Check sheet for the modelled part. Datum: model origin and axes. Units: mm. Round coordinates to 2 decimals unless told otherwise and drop trailing zeros. Order: outer loops, then holes, each group sorted by start corner. A loop starts at its lowest first (then second) coordinate and runs counter-clockwise, first axis right, second up.
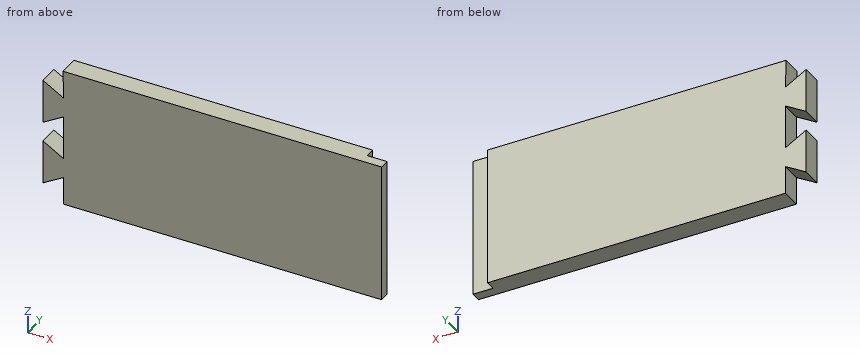
```python
from build123d import *

# Parameters (mm, degrees)
F0_W     = 340
F0_H     = 140
F1_DEPTH = 20
F4_DEPTH = 20
F2_W     = 10
F2_H     = 140
F5_DEPTH = 20


with BuildPart() as f1:
    # F0 (on Front) → F1 (new body)
    with BuildSketch(Plane.XZ):
        Rectangle(F0_W, F0_H)
    extrude(amount=F1_DEPTH)

    # F3 (on face) → F4 (cut)
    with BuildSketch(Plane(origin=(0, 0, 0), x_dir=(-1, 0, 0), z_dir=(0, 1, 0))):
        Polygon((149.1751, -41.837405), (149.1751, -70), (150, -70), (170, -70), (170, -54.026762), align=None)
        Polygon((170, 54.026762), (170, 70), (150, 70), (149.1751, 41.837405), align=None)
        Polygon((170, 0), (170, 9.882683), (149.1751, 22.07204), (149.1751, -22.07204), (170, -9.882683), align=None)
    extrude(amount=-F4_DEPTH, mode=Mode.SUBTRACT)

    # F2 (on face) → F5 (cut)
    with BuildSketch(Plane.YZ.offset(170)):
        with Locations((-5, 0)):
            Rectangle(F2_W, F2_H)
    extrude(amount=-F5_DEPTH, mode=Mode.SUBTRACT)


solid = f1.part
```
Item 1: Sectioned sample at B-B (y = -7). Record the cut outline in (x, z), and give its area (3 significant figures).
Answer:
outline: (-170, -54.03) - (-149.18, -41.84) - (-149.18, -70) - (150, -70) - (150, 70) - (-150, 70) - (-149.18, 41.84) - (-170, 54.03) - (-170, 9.88) - (-149.18, 22.07) - (-149.18, -22.07) - (-170, -9.88) - close
area: 43,200 mm2
Item 2: Sectioned sample at A-A (z = -13.5). Record the cut outline in (x, y).
Answer:
outline: (-170, -20) - (-163.82, -20) - (-163.82, 0) - (-170, 0) - close; (-149.18, -20) - (170, -20) - (170, -10) - (150, -10) - (150, 0) - (-149.18, 0) - close
Item 3: Go/stop test with a flat-tipped pin: P1, Ø6, axis at y = -9.5, z = 3, coming from the -X side. Record where the tip stops, or that it passes through.
Answer:
P1: stops at x = -149.18
Item 4: Sectioned sample at D-D (z = -46). Record the cut outline in (x, y), and give its area (3 significant figures).
Answer:
outline: (-170, -20) - (-156.29, -20) - (-156.29, 0) - (-170, 0) - close; (-149.18, -20) - (170, -20) - (170, -10) - (150, -10) - (150, 0) - (-149.18, 0) - close
area: 6,460 mm2
Item 5: Scan lines: line 1 along X through (y, z) = (-0.75, 7.5); line 2 along X through (y, z) = (-6, 21); line 3 along X through (y, z) = (-14, 43). Record each from-to range of solid material in increasing order.
Answer:
line 1: x = -149.18 to 150
line 2: x = -170 to -151.01, -149.18 to 150
line 3: x = -170 to -151.16, -149.21 to 170
Item 6: Sectioned sample at C-C (z = 25.5). Record the cut outline in (x, y), and give its area (3 significant figures).
Answer:
outline: (-170, -20) - (170, -20) - (170, -10) - (150, -10) - (150, 0) - (-170, 0) - close
area: 6,600 mm2
